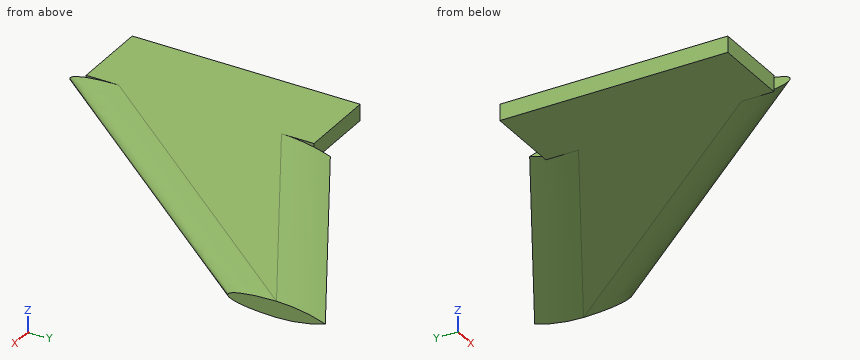
from build123d import *

# Parameters (mm, degrees)
BOSS_EXTRUDE1_DEPTH = 5
CUT_EXTRUDE2_DEPTH  = 120.505652991
CUT_EXTRUDE3_DEPTH  = 87.577477123
SKETCH6_R           = 15.9
CUT_EXTRUDE7_DEPTH  = 126.900754709


with BuildPart() as part:
    # Sketch1 → Boss-Extrude1 (new body)
    with BuildSketch(Plane.XY):
        Polygon((0, 0), (0, 70), (25, 70), (25, 75), (101, 118.517979035), (101, 88.517979035), (25, -5), (25, 0), align=None)
    extrude(amount=BOSS_EXTRUDE1_DEPTH)

    # Sketch4 → Cut-Extrude2 (cut, along a direction that is not the sketch's normal)
    with BuildSketch(Plane(origin=(101, 0, 0), x_dir=(0, 0, -1), z_dir=(1, 0, 0))):
        with BuildLine():
            Line((0, 88.517979035), (0, 103.517979035))
            add(Edge.make_bspline(
                [(-2.5, 88.517979035), (0, 88.517979035), (0, 103.517979035)],
                knots=[6.283185307, 6.283185307, 6.283185307, 7.853981634, 7.853981634, 7.853981634], degree=2, weights=[1, 0.707106781, 1]))
            Line((-2.5, 88.517979035), (0, 88.517979035))
        make_face()
        with BuildLine():
            add(Edge.make_bspline(
                [(-5, 103.517979035), (-5, 88.517979035), (-2.5, 88.517979035)],
                knots=[4.71238898, 4.71238898, 4.71238898, 6.283185307, 6.283185307, 6.283185307], degree=2, weights=[1, 0.707106781, 1]))
            Line((-5, 103.517979035), (-5, 88.517979035))
            Line((-5, 88.517979035), (-2.5, 88.517979035))
        make_face()
    extrude(amount=-CUT_EXTRUDE2_DEPTH, dir=(0.6306758074312901, 0.7760464070665428, 0), mode=Mode.SUBTRACT)

    # Sketch5 → Cut-Extrude3 (cut, along a direction that is not the sketch's normal)
    with BuildSketch(Plane(origin=(101, 0, 0), x_dir=(0, 0, -1), z_dir=(1, 0, 0))):
        with BuildLine():
            ThreePointArc((-2.5, 118.517979035), (-0.629281023, 111.121432198), (0, 103.517979035))
            Line((0, 103.517979035), (0, 118.517979035))
            Line((0, 118.517979035), (-2.5, 118.517979035))
        make_face()
        with BuildLine():
            Line((-5, 118.517979035), (-5, 103.517979035))
            ThreePointArc((-5, 103.517979035), (-4.370718977, 111.121432198), (-2.5, 118.517979035))
            Line((-2.5, 118.517979035), (-5, 118.517979035))
        make_face()
    extrude(amount=-CUT_EXTRUDE3_DEPTH, dir=(0.8678030299169633, 0.4969083429234592, 0), mode=Mode.SUBTRACT)

    # Sketch6 → Cut-Extrude7 (cut, through all)
    with BuildSketch(Plane(origin=(0, 70, 0), x_dir=(1, 0, 0), z_dir=(0, 1, 0))):
        with Locations((-14.6, -2.5)):
            Circle(SKETCH6_R)
    extrude(amount=-CUT_EXTRUDE7_DEPTH, mode=Mode.SUBTRACT)


solid = part.part
For this review, take the finished solid that the model builds, in its own axes (mm). Give positions to 0.01 mm unless a question says otherwise; leave off trailing zeros. Loops run counter-clockwise (first coordinate to the right, second up) from the corner with the lowest first, then second, coordinate; pieces in that order, holes last. Notation, with made-up numbers: M -15.5,52 L 11.5,52 A25 cw 11.5,90 Z; hole C 6,69 d11. An arc over 180 degrees is marked long. Answer as a JSON object with one key per item and string values. Group by question number.
Q1. Insertion check: P1, Ø2, axis at y = 73.5, z = 2, coming from the -X side; P2, Ø4, axis at x = 44.5, y = 16.5, coming from the -Z side; P3, Ø2.5, axis at x = 14, z = 3.5, coming from the -Y side. Each pin has a flat end and moves straight along its axis. Give the tip position at first contact, or say it passes through.
Q2. Add section A-A on x = 8. Give the boundary of the cut face in (y, z), and give its area (3 significant figures).
Q3. For probe 1 along Z at (x, y) = (83, 79.5); probe 2 along Y at (x, z) = (12, 1.8); probe 3 along Z at (x, y) = (76, 64), list the stretches that pass through material, from the lowest coordinate up. Write a range as [from, to].
Checked values:
{
 "1": {"P1": "x = 25", "P2": "z = 1.76", "P3": "y = 0"},
 "2": {"outline": "M 0,0 L 70,0 L 70,5 L 0,5 Z", "area": "350 mm²"},
 "3": {"probe 1": "[0.02, 4.98]", "probe 2": "[0, 70]", "probe 3": "[0.47, 4.53]"}
}
